Autodesk Inventor part; units mm, degrees
ref_plane "YZ Plane" through (0, 0, 0) normal (1, 0, 0) x (0, 1, 0)
ref_plane "XZ Plane" through (0, 0, 0) normal (0, 1, 0) x (-1, 0, 0)
ref_plane "XY Plane" through (0, 0, 0) normal (0, 0, 1) x (1, 0, 0)
sketch "Skizze1" plane through (0, 0, 0) normal (0, 1, 0) x (-1, 0, 0)
  circle A0 centre (0, 0) radius 1.6
  circle A1 centre (0, 0) radius 3.5
  line L0 (-1.5, 3.1623) -> (-1.5, 48.5)
  line L1 (-1.5, 48.5) -> (1.5, 48.5)
  line L2 (1.5, 48.5) -> (1.5, 3.1623)
  line L3 (0, -67.9) -> (0, 67.9) construction
  line L4 (-40, 0) -> (12.5, 0) construction
  line L5 (-5, 45.5) -> (5, 45.5)
  line L6 (5, 45.5) -> (5, 48.5)
  line L7 (5, 48.5) -> (-5, 48.5)
  line L8 (-5, 48.5) -> (-5, 45.5)
  line L9 (-5, 45.5) -> (5, 48.5) construction
  line L10 (5, 45.5) -> (-5, 48.5) construction
  line L11 (-1.5, -3.1623) -> (-1.5, -48.5)
  line L12 (-1.5, -48.5) -> (1.5, -48.5)
  line L13 (1.5, -48.5) -> (1.5, -3.1623)
  line L14 (-5, -45.5) -> (5, -45.5)
  line L15 (5, -45.5) -> (5, -48.5)
  line L16 (5, -48.5) -> (-5, -48.5)
  line L17 (-5, -48.5) -> (-5, -45.5)
  line L18 (-5, -45.5) -> (5, -48.5) construction
  line L19 (5, -45.5) -> (-5, -48.5) construction
  line L20 (-3.1623, 1.5) -> (-32.5, 1.5)
  line L21 (-32.5, 1.5) -> (-32.5, -1.5)
  line L22 (-32.5, -1.5) -> (-3.1623, -1.5)
  line L23 (-3.1623, -1.5) -> (-3.1623, 1.5)
  point P0 (0, 47)
  point P1 (0, -47)
  point P2 (-3.1623, -1.5)
  point P3 (-1.5, -45.5)
  point P4 (1.5, -45.5)
  point P5 (1.5, -3.1623)
  point P6 (1.5, 45.5)
  point P7 (-1.5, 45.5)
  dimension "d0" = 3.2
  dimension "d1" = 7
  dimension "d2" = 3
  dimension "d3" = 48.5
  dimension "d4" = 3
  dimension "d5" = 10
  dimension "d6" = 3
  dimension "d7" = 32.5
extrude "Extrusion1" add sketch "Skizze1" along normal blind 3
mirror "Spiegeln1" about plane through (32.5, 0, 1.5) normal (1, 0, 0)
properties part number "RSP-Spacer"
CAD build for the part. Positions are in the model's coordinates, mm. A direction names the side the tool comes from. Coordinates: 2 decimals unless noted, no trailing zeros. Order: outer loops, then holes, each group sorted by start corner. A loop starts at its lowest first (then second) coordinate and runs counter-clockwise, first axis right, second up. Notation, with made-up numbers: (4.5, -34.75) -> (30.5, -34.75) arc R34 cw to (30.5, 1.25) -> close; hole circle Ø3 at (-37.5, -1.5). An arc over 180 degrees is marked (long way). Answer in a Markdown table with one row per item.
1) Band-saw the part on C-C (z = -36). List the corners of the cut face in (x, y), and give its area (3 significant figures).
Check values:
| item | result |
|---|---|
| outline | (-1.5, 0) -> (1.5, 0) -> (1.5, 3) -> (-1.5, 3) -> close; (63.5, 0) -> (66.5, 0) -> (66.5, 3) -> (63.5, 3) -> close |
| area | 18.0 mm2 |
2) Which spindle directions (+Z, -Z, +X, -X, +Y, -Y) get a long thin tool onto all of the face, cutting with end or side? Do faces 4 (the face through (5, 1, 47)), 5 (the face through (68, 1, 45.5)), 6 (the face through (5, 1, -47)). Say none if no direction does.
Check values:
| item | result |
|---|---|
| face 4 | +Z, +Y, -Y |
| face 5 | +X, +Y, -Y |
| face 6 | -Z, +Y, -Y |
3) Band-saw the part on B-B (x = 65). List the corners of the cut face in (y, z), and give its area (3 significant figures).
Check values:
| item | result |
|---|---|
| outline | (0, -48.5) -> (3, -48.5) -> (3, -1.6) -> (0, -1.6) -> close; (0, 1.6) -> (3, 1.6) -> (3, 48.5) -> (0, 48.5) -> close |
| area | 281 mm2 |
4) Band-saw the part on A-A (z = 0). List the corners of the cut face in (x, y).
Check values:
| item | result |
|---|---|
| outline | (-3.5, 0) -> (-1.6, 0) -> (-1.6, 3) -> (-3.5, 3) -> close; (1.6, 0) -> (63.4, 0) -> (63.4, 3) -> (1.6, 3) -> close; (66.6, 0) -> (68.5, 0) -> (68.5, 3) -> (66.6, 3) -> close |
5) Band-saw the part on D-D (x = 42). List the corners of the cut face in (y, z), and give its area (3 significant figures).
Check values:
| item | result |
|---|---|
| outline | (0, -1.5) -> (3, -1.5) -> (3, 1.5) -> (0, 1.5) -> close |
| area | 9.00 mm2 |
6) Mould opens along X. For faces 1 (the face through (63.5, 1, 25)), 2 (the face through (-5, 1, 47)), 3 (the face through (-3, 1, 45.5)) say: pulls with the +X half, pulls with the -X half, needs draft (parallel to the pull), parting line crosses it, or undercut.
Check values:
| item | result |
|---|---|
| face 1 | undercut |
| face 2 | pulls with the -X half |
| face 3 | needs draft |
7) Flat gauge pins, fed straight in: P1, Ø1.5, axis at y = 1.5, z = 29.5, coming from the -X side; P2, Ø0.9, axis at x = 41, y = 1.5, coming from the -Z side; P3, Ø1, axis at y = 2.5, z = -34, coming from the +X side. Where does each tip first touch, or does it go through?
Check values:
| item | result |
|---|---|
| P1 | x = -1.5 |
| P2 | z = -1.5 |
| P3 | x = 66.5 |
8) Drill centre lines: line 1 (Z direction, x = 65, y = 1); line 2 (X direction, y = 0.35, z = -5); line 3 (X direction, y = 2.65, z = 1). Where is each one in solid material? Low to high.
Check values:
| item | result |
|---|---|
| line 1 | -48.5 to -1.6, 1.6 to 48.5 |
| line 2 | -1.5 to 1.5, 63.5 to 66.5 |
| line 3 | -3.35 to -1.25, 1.25 to 63.75, 66.25 to 68.35 |
